from build123d import *

# Parameters (mm, degrees)
F0_W     = 3.5
F0_H     = 1.4879982061
F0_W_2   = 3.25
F0_H_2   = 10
F0_H_3   = 0.5193831472
F1_DEPTH = 0.5
F2_DEPTH = 5


# Not quite as in the source:
# - a feature of the source that left no trace in its solid (it failed there, or was rolled back) is left out
# - a feature names something its author has since deleted; it is built from what else it names


with BuildPart() as f1:
    # F0 (on Top) → F1 (new body)
    with BuildSketch(Plane.XY):
        with BuildLine():
            Line((-1.75, 5), (-1.75, 19.3711125132))
            ThreePointArc((-1.75, 19.3711125132), (-3.3872134677, 19.1527879152), (-5, 18.7963427294))
            Line((-5, 18.7963427294), (-5, 5))
            Line((-5, 5), (-1.75, 5))
        make_face()
        with BuildLine():
            ThreePointArc((-5, 18.7963427294), (-3.3872134677, 19.1527879152), (-1.75, 19.3711125132))
            Line((-1.75, 19.3711125132), (-1.75, 20.8591107193))
            Line((-1.75, 20.8591107193), (-5, 20.8591107193))
            Line((-5, 20.8591107193), (-5, 18.7963427294))
        make_face()
        with Locations((0, 20.1151116163)):
            Rectangle(F0_W, F0_H)
        with BuildLine():
            Line((-5, 5), (-5, 18.7963427294))
            ThreePointArc((-5, 18.7963427294), (-13.7532268941, 13.7532268941), (-18.7963427294, 5))
            Line((-18.7963427294, 5), (-5, 5))
        make_face()
        with BuildLine():
            ThreePointArc((-18.7963427294, 5), (-13.7532268941, 13.7532268941), (-5, 18.7963427294))
            Line((-5, 18.7963427294), (-5, 20.8591107193))
            ThreePointArc((-5, 20.8591107193), (-15.1674404565, 15.1674404565), (-20.8591107193, 5))
            Line((-20.8591107193, 5), (-18.7963427294, 5))
        make_face()
        with Locations((-3.375, 0)):
            Rectangle(F0_W_2, F0_H_2)
        with Locations((0, 21.1188022929)):
            Rectangle(F0_W, F0_H_3)
        with BuildLine():
            Line((-5, 20.8591107193), (-1.75, 20.8591107193))
            Line((-1.75, 20.8591107193), (-1.75, 21.3784938665))
            ThreePointArc((-1.75, 21.3784938665), (-3.3849763239, 21.1812283706), (-5, 20.8591107193))
        make_face()
        with BuildLine():
            ThreePointArc((5, 18.7963427294), (3.3872134677, 19.1527879152), (1.75, 19.3711125132))
            Line((1.75, 19.3711125132), (1.75, 5))
            Line((1.75, 5), (5, 5))
            Line((5, 5), (5, 18.7963427294))
        make_face()
        with BuildLine():
            Line((1.75, 20.8591107193), (1.75, 19.3711125132))
            ThreePointArc((1.75, 19.3711125132), (3.3872134677, 19.1527879152), (5, 18.7963427294))
            Line((5, 18.7963427294), (5, 20.8591107193))
            Line((5, 20.8591107193), (1.75, 20.8591107193))
        make_face()
        with BuildLine():
            Line((-5, 5), (-18.7963427294, 5))
            ThreePointArc((-18.7963427294, 5), (-19.45, 0), (-18.7963427294, -5))
            Line((-18.7963427294, -5), (-5, -5))
            Line((-5, -5), (-5, 5))
        make_face()
        with BuildLine():
            ThreePointArc((-18.7963427294, -5), (-19.45, 0), (-18.7963427294, 5))
            Line((-18.7963427294, 5), (-20.8591107193, 5))
            Line((-20.8591107193, 5), (-20.8591107193, -5))
            Line((-20.8591107193, -5), (-18.7963427294, -5))
        make_face()
        with Locations((3.375, 0)):
            Rectangle(F0_W_2, F0_H_2)
        with BuildLine():
            Line((-1.75, -19.3711125132), (-1.75, -5))
            Line((-1.75, -5), (-5, -5))
            Line((-5, -5), (-5, -18.7963427294))
            ThreePointArc((-5, -18.7963427294), (-3.3872134677, -19.1527879152), (-1.75, -19.3711125132))
        make_face()
        with BuildLine():
            Line((1.75, 21.3784938665), (1.75, 20.8591107193))
            Line((1.75, 20.8591107193), (5, 20.8591107193))
            ThreePointArc((5, 20.8591107193), (3.3849763239, 21.1812283706), (1.75, 21.3784938665))
        make_face()
        with BuildLine():
            ThreePointArc((1.75, 21.3784938665), (0, 21.45), (-1.75, 21.3784938665))
            Line((-1.75, 21.3784938665), (1.75, 21.3784938665))
        make_face()
        with BuildLine():
            ThreePointArc((18.7963427294, 5), (13.7532268941, 13.7532268941), (5, 18.7963427294))
            Line((5, 18.7963427294), (5, 5))
            Line((5, 5), (18.7963427294, 5))
        make_face()
        with BuildLine():
            Line((5, 20.8591107193), (5, 18.7963427294))
            ThreePointArc((5, 18.7963427294), (13.7532268941, 13.7532268941), (18.7963427294, 5))
            Line((18.7963427294, 5), (20.8591107193, 5))
            ThreePointArc((20.8591107193, 5), (15.1674404565, 15.1674404565), (5, 20.8591107193))
        make_face()
        with BuildLine():
            Line((-5, -5), (-18.7963427294, -5))
            ThreePointArc((-18.7963427294, -5), (-13.7532268941, -13.7532268941), (-5, -18.7963427294))
            Line((-5, -18.7963427294), (-5, -5))
        make_face()
        with BuildLine():
            ThreePointArc((-5, -18.7963427294), (-13.7532268941, -13.7532268941), (-18.7963427294, -5))
            Line((-18.7963427294, -5), (-20.8591107193, -5))
            ThreePointArc((-20.8591107193, -5), (-15.1674404565, -15.1674404565), (-5, -20.8591107193))
            Line((-5, -20.8591107193), (-5, -18.7963427294))
        make_face()
        with BuildLine():
            Line((-20.8591107193, -5), (-20.8591107193, 5))
            ThreePointArc((-20.8591107193, 5), (-21.45, 0), (-20.8591107193, -5))
        make_face()
        with BuildLine():
            Line((18.7963427294, 5), (5, 5))
            Line((5, 5), (5, -5))
            Line((5, -5), (18.7963427294, -5))
            ThreePointArc((18.7963427294, -5), (19.45, 0), (18.7963427294, 5))
        make_face()
        with BuildLine():
            Line((5, -5), (1.75, -5))
            Line((1.75, -5), (1.75, -19.3711125132))
            ThreePointArc((1.75, -19.3711125132), (3.3872134677, -19.1527879152), (5, -18.7963427294))
            Line((5, -18.7963427294), (5, -5))
        make_face()
        with BuildLine():
            Line((-1.75, -20.8591107193), (-1.75, -19.3711125132))
            ThreePointArc((-1.75, -19.3711125132), (-3.3872134677, -19.1527879152), (-5, -18.7963427294))
            Line((-5, -18.7963427294), (-5, -20.8591107193))
            Line((-5, -20.8591107193), (-1.75, -20.8591107193))
        make_face()
        with Locations((0, -20.1151116163)):
            Rectangle(F0_W, F0_H)
        with BuildLine():
            Line((20.8591107193, 5), (18.7963427294, 5))
            ThreePointArc((18.7963427294, 5), (19.45, 0), (18.7963427294, -5))
            Line((18.7963427294, -5), (20.8591107193, -5))
            Line((20.8591107193, -5), (20.8591107193, 5))
        make_face()
        with BuildLine():
            Line((18.7963427294, -5), (5, -5))
            Line((5, -5), (5, -18.7963427294))
            ThreePointArc((5, -18.7963427294), (13.7532268941, -13.7532268941), (18.7963427294, -5))
        make_face()
        with BuildLine():
            ThreePointArc((5, -18.7963427294), (3.3872134677, -19.1527879152), (1.75, -19.3711125132))
            Line((1.75, -19.3711125132), (1.75, -20.8591107193))
            Line((1.75, -20.8591107193), (5, -20.8591107193))
            Line((5, -20.8591107193), (5, -18.7963427294))
        make_face()
        with BuildLine():
            Line((-1.75, -21.3784938665), (-1.75, -20.8591107193))
            Line((-1.75, -20.8591107193), (-5, -20.8591107193))
            ThreePointArc((-5, -20.8591107193), (-3.3849763239, -21.1812283706), (-1.75, -21.3784938665))
        make_face()
        with Locations((0, -21.1188022929)):
            Rectangle(F0_W, F0_H_3)
        with BuildLine():
            ThreePointArc((21.45, 0), (21.3017654776, 2.5173969761), (20.8591107193, 5))
            Line((20.8591107193, 5), (20.8591107193, -5))
            ThreePointArc((20.8591107193, -5), (21.3017654776, -2.5173969761), (21.45, 0))
        make_face()
        with BuildLine():
            Line((20.8591107193, -5), (18.7963427294, -5))
            ThreePointArc((18.7963427294, -5), (13.7532268941, -13.7532268941), (5, -18.7963427294))
            Line((5, -18.7963427294), (5, -20.8591107193))
            ThreePointArc((5, -20.8591107193), (15.1674404565, -15.1674404565), (20.8591107193, -5))
        make_face()
        with BuildLine():
            Line((5, -20.8591107193), (1.75, -20.8591107193))
            Line((1.75, -20.8591107193), (1.75, -21.3784938665))
            ThreePointArc((1.75, -21.3784938665), (3.3849763239, -21.1812283706), (5, -20.8591107193))
        make_face()
        with BuildLine():
            Line((1.75, -21.3784938665), (-1.75, -21.3784938665))
            ThreePointArc((-1.75, -21.3784938665), (0, -21.45), (1.75, -21.3784938665))
        make_face()
    extrude(amount=F1_DEPTH)

    # F0 (on Top) → F2 (join)
    with BuildSketch(Plane.XY):
        with BuildLine():
            ThreePointArc((-5, 18.7963427294), (-3.3872134677, 19.1527879152), (-1.75, 19.3711125132))
            Line((-1.75, 19.3711125132), (-1.75, 20.8591107193))
            Line((-1.75, 20.8591107193), (-5, 20.8591107193))
            Line((-5, 20.8591107193), (-5, 18.7963427294))
        make_face()
        with Locations((0, 20.1151116163)):
            Rectangle(F0_W, F0_H)
        with Locations((0, 21.1188022929)):
            Rectangle(F0_W, F0_H_3)
        with BuildLine():
            Line((-5, 20.8591107193), (-1.75, 20.8591107193))
            Line((-1.75, 20.8591107193), (-1.75, 21.3784938665))
            ThreePointArc((-1.75, 21.3784938665), (-3.3849763239, 21.1812283706), (-5, 20.8591107193))
        make_face()
        with BuildLine():
            Line((1.75, 20.8591107193), (1.75, 19.3711125132))
            ThreePointArc((1.75, 19.3711125132), (3.3872134677, 19.1527879152), (5, 18.7963427294))
            Line((5, 18.7963427294), (5, 20.8591107193))
            Line((5, 20.8591107193), (1.75, 20.8591107193))
        make_face()
        with BuildLine():
            ThreePointArc((-18.7963427294, -5), (-19.45, 0), (-18.7963427294, 5))
            Line((-18.7963427294, 5), (-20.8591107193, 5))
            Line((-20.8591107193, 5), (-20.8591107193, -5))
            Line((-20.8591107193, -5), (-18.7963427294, -5))
        make_face()
        with BuildLine():
            Line((1.75, 21.3784938665), (1.75, 20.8591107193))
            Line((1.75, 20.8591107193), (5, 20.8591107193))
            ThreePointArc((5, 20.8591107193), (3.3849763239, 21.1812283706), (1.75, 21.3784938665))
        make_face()
        with BuildLine():
            ThreePointArc((1.75, 21.3784938665), (0, 21.45), (-1.75, 21.3784938665))
            Line((-1.75, 21.3784938665), (1.75, 21.3784938665))
        make_face()
        with BuildLine():
            Line((-20.8591107193, -5), (-20.8591107193, 5))
            ThreePointArc((-20.8591107193, 5), (-21.45, 0), (-20.8591107193, -5))
        make_face()
        with BuildLine():
            Line((-1.75, -20.8591107193), (-1.75, -19.3711125132))
            ThreePointArc((-1.75, -19.3711125132), (-3.3872134677, -19.1527879152), (-5, -18.7963427294))
            Line((-5, -18.7963427294), (-5, -20.8591107193))
            Line((-5, -20.8591107193), (-1.75, -20.8591107193))
        make_face()
        with Locations((0, -20.1151116163)):
            Rectangle(F0_W, F0_H)
        with BuildLine():
            Line((20.8591107193, 5), (18.7963427294, 5))
            ThreePointArc((18.7963427294, 5), (19.45, 0), (18.7963427294, -5))
            Line((18.7963427294, -5), (20.8591107193, -5))
            Line((20.8591107193, -5), (20.8591107193, 5))
        make_face()
        with BuildLine():
            ThreePointArc((5, -18.7963427294), (3.3872134677, -19.1527879152), (1.75, -19.3711125132))
            Line((1.75, -19.3711125132), (1.75, -20.8591107193))
            Line((1.75, -20.8591107193), (5, -20.8591107193))
            Line((5, -20.8591107193), (5, -18.7963427294))
        make_face()
        with BuildLine():
            Line((-1.75, -21.3784938665), (-1.75, -20.8591107193))
            Line((-1.75, -20.8591107193), (-5, -20.8591107193))
            ThreePointArc((-5, -20.8591107193), (-3.3849763239, -21.1812283706), (-1.75, -21.3784938665))
        make_face()
        with Locations((0, -21.1188022929)):
            Rectangle(F0_W, F0_H_3)
        with BuildLine():
            ThreePointArc((21.45, 0), (21.3017654776, 2.5173969761), (20.8591107193, 5))
            Line((20.8591107193, 5), (20.8591107193, -5))
            ThreePointArc((20.8591107193, -5), (21.3017654776, -2.5173969761), (21.45, 0))
        make_face()
        with BuildLine():
            Line((5, -20.8591107193), (1.75, -20.8591107193))
            Line((1.75, -20.8591107193), (1.75, -21.3784938665))
            ThreePointArc((1.75, -21.3784938665), (3.3849763239, -21.1812283706), (5, -20.8591107193))
        make_face()
        with BuildLine():
            Line((1.75, -21.3784938665), (-1.75, -21.3784938665))
            ThreePointArc((-1.75, -21.3784938665), (0, -21.45), (1.75, -21.3784938665))
        make_face()
    extrude(amount=F2_DEPTH)


solid = f1.part
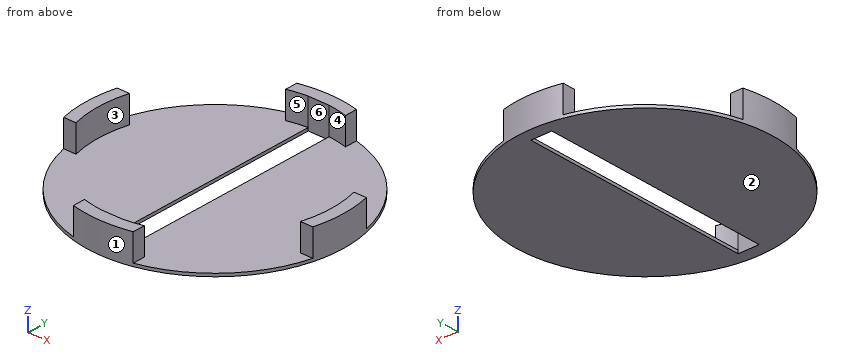
Input: part model. Units: mm. Frame: model coordinates. Face numbers are marked on the shaded views. A direction names the side the tool comes from. Give positions to 0.01 mm unless a question says otherwise; leave off trailing zeros. Write each loop counter-clockwise with the first axis right and the second up, starting at its lowest first coordinate (ties: lowest second). Pieces come first, ordered by that corner, then holes.
Q1. Pull-direction query (Y, two-part tool) for the marked faces 1, 2, 3 and 4; classes: pulls with the +Y half, pulls with the -Y half, needs draft (parallel to the pull), parting line crosses it, or undercut.
Q2. First-contact query: P1, Ø1, axis at x = 20, z = 2.5, coming from the +Y side; P2, Ø1.7, axis at y = 20.5, z = 3, coming from the +X side; P3, Ø15.5, axis at x = 6.5, y = 5, coming from the +Z side; P4, Ø1, axis at x = -6.5, z = 3, coming from the -Y side. Flat tips, straight axial feed; report the tip coordinate or a pass-through.
Q3. Section C-C, the plane y = 0. Output: boundary loops of the cut face in (x, z).
Q4. Section A-A, the plane z = 2.2. Output: boundary loops of the cut face in (x, y).
Q5. Material intervals for probe 1 along Z at (x, y) = (15.5, 6); probe 2 along X at (y, z) = (-20, 4.15); probe 3 along X at (y, z) = (-2, 3.4), sorted ascending.
Q6. Section D-D, the plane y = 13.5. Output: boundary loops of the cut face in (x, z), plus the area to 3 significant figures.
Q7. Set-up query: the marked faces 5 and 6. Return all of +Z, -Z, +X, -X, +Y, -Y with unobstructed straight access to the full face (end or side cutting, diameter ignored); none if empty.
Q8. Section B-B, the plane x = 0. Output: boundary loops of the cut face in (y, z), plus the area to 3 significant figures.
Filled in:
1. face 1: parting line crosses it
1. face 2: needs draft
1. face 3: undercut
1. face 4: undercut
2. P1: stops at y = 5
2. P2: stops at x = 5
2. P3: stops at z = 0.5
2. P4: passes through
3. outline: (-21.45, 0) - (-1.75, 0) - (-1.75, 0.5) - (-19.45, 0.5) - (-19.45, 5) - (-21.45, 5) - close; (1.75, 0) - (21.45, 0) - (21.45, 5) - (19.45, 5) - (19.45, 0.5) - (1.75, 0.5) - close
4. outline: (-20.86, -5) - (-18.8, -5) arc R19.45 cw to (-18.8, 5) - (-20.86, 5) arc R21.45 ccw to start; (-5, -20.86) arc R21.45 ccw to (5, -20.86) - (5, -18.8) arc R19.45 cw to (1.75, -19.37) - (-1.75, -19.37) arc R19.45 cw to (-5, -18.8) - close; (-5, 18.8) arc R19.45 cw to (-1.75, 19.37) - (1.75, 19.37) arc R19.45 cw to (5, 18.8) - (5, 20.86) arc R21.45 ccw to (-5, 20.86) - close; (18.8, -5) - (20.86, -5) arc R21.45 ccw to (20.86, 5) - (18.8, 5) arc R19.45 cw to start
5. probe 1: z = 0 to 0.5
5. probe 2: x = -5 to 5
5. probe 3: x = -21.36 to -19.35, 19.35 to 21.36
6. outline: (-16.67, 0) - (-1.75, 0) - (-1.75, 0.5) - (-16.67, 0.5) - close; (1.75, 0) - (16.67, 0) - (16.67, 0.5) - (1.75, 0.5) - close
6. area: 14.9 mm2
7. face 5: +Z
7. face 6: +Z, -Z
8. outline: (-21.45, 0) - (-19.37, 0) - (-19.37, 5) - (-21.45, 5) - close; (19.37, 0) - (21.45, 0) - (21.45, 5) - (19.37, 5) - close
8. area: 20.8 mm2
